The model under review builds one solid part; all positions refer to its coordinate system, in mm. Give positions to 0.01 mm unless a question says otherwise; leave off trailing zeros. Order: outer loops, then holes, each group sorted by start corner. A loop starts at its lowest first (then second) coordinate and runs counter-clockwise, first axis right, second up. Notation, with made-up numbers: M 48.25,9.25 L 70.25,9.25 A29 ccw 70.25,39.25 Z; hole C 52.25,-20.75 d5. An arc over 180 degrees is marked long. One line per question, with ' | ' between items. Start each with the question number.
1. We need section C-C on y = -9. Write out the cut boundary in (x, z), then the cut area to 3 significant figures.
2. The part is to be moulded in two halves that separate along Z. For faces 1 (the face through (-11, 17, 3)), 2 (the face through (-9.76, 0.22, -2.17)), 3 (the face through (11.172, 0.224, 7.123)), say which applies: +Z half, -Z half, draft (parallel to the pull), parting line (faces both ways), or undercut.
3. We need section A-A on z = 0. Write out the cut boundary in (x, y).
4. Wall thickness on L1, parallel to X at y = 7.5, z = 0; L2, parallel to X at y = -0.5, z = -7.5; L3, parallel to Z at x = 8.5, y = 5: over which ranges is each line inside the solid? List them lowest first.
5. We need section B-B on x = 0. Write out the cut boundary in (y, z).
6. Insertion check: P1, Ø6, axis at x = 7, y = 5.5, coming from the +Z side; P2, Ø1.5, axis at y = 4.5, z = -3, coming from the -X side; P3, Ø6, axis at x = 10.5, y = 11.5, coming from the +Z side. Each pin has a flat end and moves straight along its axis. Give the tip position at first contact, or say it passes through.
```python
from build123d import *

# Parameters (mm, degrees)
F0_W     = 34
F0_H     = 3.25
F2_SIZE2 = 0.5773502692
F2_SIZE  = 1
F3_SIZE2 = 0.5
F3_SIZE  = 0.5
F4_R     = 1


with BuildPart() as f1:
    # F0 (on Right) → F1 (revolve)
    with BuildSketch(Plane.YZ):
        with Locations((0, 11.625)):
            Rectangle(F0_W, F0_H)
    revolve(axis=Axis((0, 0.0117017189, 0), (0, 1, 0)))

    # F2
    f2_edges = [f1.edges().sort_by_distance(p)[0] for p in [
        (0, -17, -10),
        (0, 17, -10),
    ]]
    f2_side = f1.faces().sort_by_distance((0, 0, -10))[0]
    chamfer(f2_edges, length=F2_SIZE, length2=F2_SIZE2, reference=f2_side)

    # F3
    f3_edges = [f1.edges().sort_by_distance(p)[0] for p in [
        (0, -17, -10.57735),
        (0, 17, -10.57735),
    ]]
    chamfer(f3_edges, length=F3_SIZE, length2=F3_SIZE2)

    # F4
    f4_edges = [f1.edges().sort_by_distance(p)[0] for p in [
        (0, 17, -13.25),
        (0, -17, -13.25),
    ]]
    fillet(f4_edges, radius=F4_R)


solid = f1.part
```
Entries:
1) outline: C 0,0 d26.5; hole C 0,0 d20 | area: 237 mm^2
2) face 1: draft | face 2: undercut | face 3: parting line
3) outline: M -13.25,-16 A1 ccw -12.25,-17 L -11.08,-17 L -10.33,-16.57 L -10,-16 L -10,16 L -10.33,16.57 L -11.08,17 L -12.25,17 A1 ccw -13.25,16 Z; M 10,-16 L 10.33,-16.57 L 11.08,-17 L 12.25,-17 A1 ccw 13.25,-16 L 13.25,16 A1 ccw 12.25,17 L 11.08,17 L 10.33,16.57 L 10,16 Z
4) L1: x = -13.25 to -10, 10 to 13.25 | L2: x = -10.92 to -6.61, 6.61 to 10.92 | L3: z = -10.16 to -5.27, 5.27 to 10.16
5) outline: M -17,-12.25 A1 ccw -16,-13.25 L 16,-13.25 A1 ccw 17,-12.25 L 17,-11.08 L 16.57,-10.33 L 16,-10 L -16,-10 L -16.57,-10.33 L -17,-11.08 Z; M -17,11.08 L -16.57,10.33 L -16,10 L 16,10 L 16.57,10.33 L 17,11.08 L 17,12.25 A1 ccw 16,13.25 L -16,13.25 A1 ccw -17,12.25 Z
6) P1: stops at z = 12.63 | P2: stops at x = -13.06 | P3: stops at z = 10.92
